For this review, use the dimensioned drawing (mm, ordinates from the lowest corner) and the shaded views. A direction names the side the tool comes from. Coordinates: 2 decimals unless noted, no trailing zeros. Loops run counter-clockwise (first coordinate to the right, second up) from the corner with the lowest first, then second, coordinate; pieces in that order, holes last. Notation, with made-up numbers: (52, -16) - (57, -16) arc R24 cw to (57, -1) - close; hole circle Ø8 at (63.5, 48). An arc over 180 degrees is marked (long way). Answer in a Markdown table with one row per item. Add a question column.
(1) We need section C-C, the plane z = 22. Write out the cut boundary in (x, y).
(2) We need section A-A, the plane z = 13.5. Write out the cut boundary in (x, y), plus the area to 3 significant figures.
(3) Clearance check with flat-ended pins moving along their axes: pin 1 (3 mm diameter, centred on x = 10, y = 16.5, fed in from +Z); pin 2 (3.5 mm diameter, centred on x = 13, z = 9, fed in from -Y). State where each tip first meets the part, or that it passes through.
(4) We need section D-D, the plane y = 12. Write out the cut boundary in (x, z).
(5) The part is to be moulded in two halves that separate along Y. For the marked faces 3, 4, 5 and 6, say which applies: released by +Y, released by -Y, zero draft, split by the parting line, or undercut.
(6) To check wall thickness, follow L1, parallel to X at y = 15.5, z = 10.5; L2, parallel to Y at x = 3.25, z = 14.5; L3, parallel to Z at x = 13.75, y = 2.5. State the ranges of each line that lie inside material, in increasing order. Write a range as [from, to].
(7) We need section B-B, the plane x = 10. Write out the cut boundary in (y, z).
(8) For the marked faces 1 and 2, list the 3-axis set-ups (+Z, -Z, +X, -X, +Y, -Y) from which the entire face can be reached by the end or side of a thin tool; tool diameter is ignored.
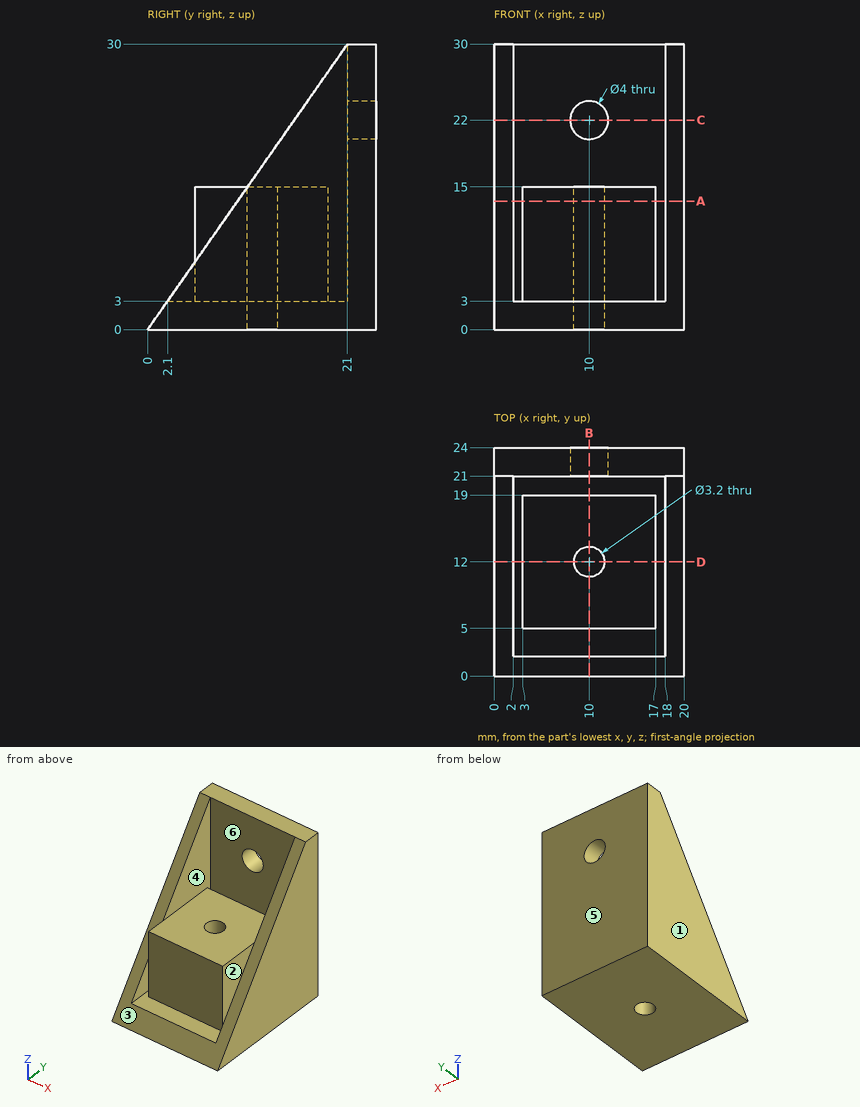
Responses:
| question | item | result |
|---|---|---|
| 1 | outline | (0, 15.4) - (2, 15.4) - (2, 21) - (8, 21) - (8, 24) - (0, 24) - close; (12, 21) - (18, 21) - (18, 15.4) - (20, 15.4) - (20, 24) - (12, 24) - close |
| 2 | outline | (0, 9.45) - (2, 9.45) - (2, 21) - (18, 21) - (18, 9.45) - (20, 9.45) - (20, 24) - (0, 24) - close; (3, 5) - (17, 5) - (17, 19) - (3, 19) - close; hole circle Ø3.2 at (10, 12) |
| 2 | area | 294 mm2 |
| 3 | pin 1 | stops at z = 15 |
| 3 | pin 2 | stops at y = 5 |
| 4 | outline | (0, 0) - (8.4, 0) - (8.4, 15) - (3, 15) - (3, 3) - (2, 3) - (2, 17.14) - (0, 17.14) - close; (11.6, 0) - (20, 0) - (20, 17.14) - (18, 17.14) - (18, 3) - (17, 3) - (17, 15) - (11.6, 15) - close |
| 5 | face 3 | released by -Y |
| 5 | face 4 | zero draft |
| 5 | face 5 | released by +Y |
| 5 | face 6 | undercut |
| 6 | L1 | x = [0, 2], [3, 17], [18, 20] |
| 6 | L2 | y = [5, 19], [21, 24] |
| 6 | L3 | z = [0, 3] |
| 7 | outline | (0, 0) - (10.4, 0) - (10.4, 15) - (5, 15) - (5, 3) - (2.1, 3) - close; (13.6, 0) - (24, 0) - (24, 20) - (21, 20) - (21, 3) - (19, 3) - (19, 15) - (13.6, 15) - close; (21, 24) - (24, 24) - (24, 30) - (21, 30) - close |
| 8 | face 1 | +Z, -Z, -X, +Y, -Y |
| 8 | face 2 | +Z, -Y |
